```python
from build123d import *

# Parameters (mm, degrees)
F0_R     = 1.2
F1_DEPTH = 1.5


with BuildPart() as f1:
    # F0 (on Front) → F1 (new body)
    with BuildSketch(Plane.XZ):
        with BuildLine():
            ThreePointArc((-1, 15), (-2.05, 13.95), (-3.1, 15))
            Line((-3.1, 15), (-6.5, 15))
            Line((-6.5, 15), (-6.5, 0))
            Line((-6.5, 0), (-6.5, -15))
            Line((-6.5, -15), (-3.1, -15))
            ThreePointArc((-3.1, -15), (-2.05, -13.95), (-1, -15))
            Line((-1, -15), (-1, -16.5))
            Line((-1, -16.5), (1, -16.5))
            Line((1, -16.5), (1, -15))
            ThreePointArc((1, -15), (2.05, -13.95), (3.1, -15))
            Line((3.1, -15), (6.5, -15))
            Line((6.5, -15), (6.5, 0))
            Line((6.5, 0), (6.5, 15))
            Line((6.5, 15), (3.1, 15))
            ThreePointArc((3.1, 15), (2.05, 13.95), (1, 15))
            Line((1, 15), (1, 16.5))
            Line((1, 16.5), (-1, 16.5))
            Line((-1, 16.5), (-1, 15))
        make_face()
        with Locations((-3.019, -7.1)):
            Circle(F0_R, mode=Mode.SUBTRACT)
        with Locations((3.019, -7.1)):
            Circle(F0_R, mode=Mode.SUBTRACT)
        with Locations((-3.019, 0)):
            Circle(F0_R, mode=Mode.SUBTRACT)
        with Locations((-3.019, 7.1)):
            Circle(F0_R, mode=Mode.SUBTRACT)
        with Locations((3.019, 0)):
            Circle(F0_R, mode=Mode.SUBTRACT)
        with Locations((3.019, 7.1)):
            Circle(F0_R, mode=Mode.SUBTRACT)
    extrude(amount=F1_DEPTH)


solid = f1.part
```
For this review, take the finished solid that the model builds, in its own axes (mm). A direction names the side the tool comes from. Round coordinates to 2 decimals unless told otherwise and drop trailing zeros. Order: outer loops, then holes, each group sorted by start corner. A loop starts at its lowest first (then second) coordinate and runs counter-clockwise, first axis right, second up.
Q1. Machinability: for faces 5 (the flat face through (1, -1, 16)), 6 (the flat face through (-5, -1, -15)), 7 (the cylindrical face through (-2.03, -0.74, 13.95)), 8 (the flat face through (-1, -1, 16)), which of the approach directions +Z, -Z, +X, -X, +Y, -Y give a long, thin tool a straight path to every point of the face, cutting with its end or side? Answer none if there is none.
Findings below:
face 5: +Z, +X, +Y, -Y
face 6: -Z, -X, +Y, -Y
face 7: +Z, +Y, -Y
face 8: +Z, -X, +Y, -Y
Q2. We need section D-D, the plane x = 1.5. Give the boundary of the cut face in (y, z), plus the area to 3 significant figures.
Findings below:
outline: (-1.5, -14.11) - (0, -14.11) - (0, 14.11) - (-1.5, 14.11) - close
area: 42.3 mm2
Q3. Mouldability with a two-part tool opening along Z and no side actions: class faces 1 (the flat face through (5, -1, 15)), 2 (the flat face through (1, -1, -16)), 3 (the cylindrical face through (2.76, -0.74, -8.27)), 4 (the flat face through (5, -1, -15)) as pulls with the +Z half, pulls with the -Z half, needs draft (parallel to the pull), parting line crosses it, or undercut.
Findings below:
face 1: pulls with the +Z half
face 2: needs draft
face 3: undercut
face 4: pulls with the -Z half
Q4. We need section A-A, the plane z = 0. Give the boundary of the cut face in (x, y).
Findings below:
outline: (-6.5, -1.5) - (-4.22, -1.5) - (-4.22, 0) - (-6.5, 0) - close; (-1.82, -1.5) - (1.82, -1.5) - (1.82, 0) - (-1.82, 0) - close; (4.22, -1.5) - (6.5, -1.5) - (6.5, 0) - (4.22, 0) - close
Q5. We need section C-C, the plane x = 5.5. Give the boundary of the cut face in (y, z), plus the area to 3 significant figures.
Findings below:
outline: (-1.5, -15) - (0, -15) - (0, 15) - (-1.5, 15) - close
area: 45.0 mm2
Q6. Insertion check: P1, Ø0.8, axis at y = -0.5, z = -15.5, coming from the -X side. The pin has a flat end and moves straight along its axis. Give the tip position at first contact, or say it passes through.
Findings below:
P1: stops at x = -1
Q7. We need section B-B, the plane y = -0.45. Give the boundary of the cut face in (x, z), plus the area to 3 significant figures.
Findings below:
outline: (-6.5, -15) - (-3.1, -15) arc R1.05 cw to (-1, -15) - (-1, -16.5) - (1, -16.5) - (1, -15) arc R1.05 cw to (3.1, -15) - (6.5, -15) - (6.5, 15) - (3.1, 15) arc R1.05 cw to (1, 15) - (1, 16.5) - (-1, 16.5) - (-1, 15) arc R1.05 cw to (-3.1, 15) - (-6.5, 15) - close; hole circle Ø2.4 at (-3.02, -7.1); hole circle Ø2.4 at (-3.02, 0); hole circle Ø2.4 at (-3.02, 7.1); hole circle Ø2.4 at (3.02, -7.1); hole circle Ø2.4 at (3.02, 0); hole circle Ø2.4 at (3.02, 7.1)
area: 362 mm2
Q8. Wall thickness on line 1 (Z direction, x = -2.5, y = -0.8); line 2 (Z direction, x = 4, y = -0.2); line 3 (X direction, y = -0.9, z = 1): over which ranges is each line inside the solid? List them lowest first.
Findings below:
line 1: z = -14.05 to -8.18, -6.02 to -1.08, 1.08 to 6.02, 8.18 to 14.05
line 2: z = -15 to -7.79, -6.41 to -0.69, 0.69 to 6.41, 7.79 to 15
line 3: x = -6.5 to -3.68, -2.36 to 2.36, 3.68 to 6.5
